```python
from build123d import *

# Parameters (mm, degrees)
EXTRUDE_1_DEPTH     = 46
SKETCH_2_R          = 3
CUT_EXTRUDE_1_DEPTH = 10
CUT_EXTRUDE_2_DEPTH = 10
FILLET_1_R          = 10


with BuildPart() as part:
    # 草图1 → 拉伸-薄壁1 (new, symmetric)
    with BuildSketch(Plane.XY):
        with BuildLine():
            Line((-15.684450605, 22.852628588), (1.315549395, 22.852628588))
            ThreePointArc((1.315549395, 22.852628588), (3.436869738, 21.973948932), (4.315549395, 19.852628588))
            Line((4.315549395, 19.852628588), (4.315549395, -12.147371412))
            ThreePointArc((4.315549395, -12.147371412), (5.194229051, -14.268691755), (7.315549395, -15.147371412))
            Line((7.315549395, -15.147371412), (17.315549395, -15.147371412))
            Line((17.315549395, -15.147371412), (17.315549395, -17.147371412))
            Line((17.315549395, -17.147371412), (7.315549395, -17.147371412))
            ThreePointArc((7.315549395, -17.147371412), (3.780015489, -15.682905318), (2.315549395, -12.147371412))
            Line((2.315549395, -12.147371412), (2.315549395, 19.852628588))
            ThreePointArc((2.315549395, 19.852628588), (2.022656176, 20.55973537), (1.315549395, 20.852628588))
            Line((1.315549395, 20.852628588), (-15.684450605, 20.852628588))
            Line((-15.684450605, 20.852628588), (-15.684450605, 22.852628588))
        make_face()
    extrude(amount=EXTRUDE_1_DEPTH, both=True)

    # 草图2 → 切除-拉伸1 (cut)
    with BuildSketch(Plane(origin=(0, -15.147371412, 0), x_dir=(1, 0, 0), z_dir=(0, 1, 0))):
        with Locations(Location((12.315549395, -38.5, 0), (0, 0, 270))):
            Circle(SKETCH_2_R)
        with Locations(Location((12.315549395, -12.5, 0), (0, 0, 270))):
            Circle(SKETCH_2_R)
        with Locations(Location((12.315549395, 12.5, 0), (0, 0, 270))):
            Circle(SKETCH_2_R)
        with Locations(Location((12.315549395, 38.5, 0), (0, 0, 270))):
            Circle(SKETCH_2_R)
    extrude(amount=-CUT_EXTRUDE_1_DEPTH, mode=Mode.SUBTRACT)

    # 草图3 → 切除-拉伸2 (cut)
    with BuildSketch(Plane(origin=(4.315549395, 0, 0), x_dir=(0, 0, -1), z_dir=(1, 0, 0))):
        with BuildLine():
            Line((-3, -7.647371412), (-3, 13.352628588))
            ThreePointArc((-3, 13.352628588), (0, 16.352628588), (3, 13.352628588))
            Line((3, 13.352628588), (3, -7.647371412))
            ThreePointArc((3, -7.647371412), (0, -10.647371412), (-3, -7.647371412))
        make_face()
    extrude(amount=-CUT_EXTRUDE_2_DEPTH, mode=Mode.SUBTRACT)

    # 圆角1
    fillet_1_edges = [part.edges().sort_by_distance(p)[0] for p in [
        (-15.684450605, 21.852628588, -46),
        (-15.684450605, 21.852628588, 46),
    ]]
    fillet(fillet_1_edges, radius=FILLET_1_R)


solid = part.part
```
CAD build for the part. Positions are in the model's coordinates, mm. A direction names the side the tool comes from. Round coordinates to 2 decimals unless told otherwise and drop trailing zeros. Order: outer loops, then holes, each group sorted by start corner. A loop starts at its lowest first (then second) coordinate and runs counter-clockwise, first axis right, second up.
Q1. Two-plate mould, pull along Z, no slides. Class faces 4 (the flat face through (12, -15.147, 1)), 5 (the cylindrical face through (-12.833, 21.867, 42.993)), 6 (the cylindrical face through (3.33, 16.35, 0.07)), 7 (the flat face through (3, 3, -3)): pulls with the +Z half, pulls with the -Z half, needs draft (parallel to the pull), parting line crosses it, or undercut.
Q2. Slice it at D-D (y = 17.5). Write the cut outline in (x, z).
Q3. Slice it at A-A (z = 12.5). Write the cut outline in (x, y).
Q4. Slice it at B-B (y = -0.5). Write the cut outline in (x, z), and give its area (3 significant figures).
Q5. Wall check: L1, parallel to X at y = 18.5, z = -35.5; L2, parallel to Y at x = 9, z = -34; L3, parallel to Y at x = 0.5, z = -5. Give the ranges that are in metal, low to high.
Q6. Which spindle directions (+Z, -Z, +X, -X, +Y, -Y) get a long thin tool onto all of the face, cutting with end or side? Do faces 1 (the flat face through (3, 3, 3)), 2 (the flat face through (2.316, 4, 11)), 3 (the cylindrical face through (12.4, -16.1, -41.5)). Say none if no direction does.
Q7. Drop flat-ended pins along their axis: pin 1 (13.5 mm diameter, centred on x = -3, z = 4.5, fed in from -Y); pin 2 (6 mm diameter, centred on x = 13, z = 12, fed in from +Y); pin 3 (8 mm diameter, centred on y = 15.5, z = -6.5, fed in from -X). Give the stop position or say it passes through.
Q8. Slice it at C-C (z = 0). Write the cut outline in (x, y).
Results below:
1. face 4: needs draft
1. face 5: pulls with the +Z half
1. face 6: undercut
1. face 7: undercut
2. outline: (2.32, -46) - (4.32, -46) - (4.32, 46) - (2.32, 46) - close
3. outline: (-15.68, 20.85) - (1.32, 20.85) arc R1 cw to (2.32, 19.85) - (2.32, -12.15) arc R5 ccw to (7.32, -17.15) - (9.32, -17.15) - (9.32, -15.15) - (7.32, -15.15) arc R3 cw to (4.32, -12.15) - (4.32, 19.85) arc R3 ccw to (1.32, 22.85) - (-15.68, 22.85) - close; (15.32, -17.15) - (17.32, -17.15) - (17.32, -15.15) - (15.32, -15.15) - close
4. outline: (2.32, -46) - (4.32, -46) - (4.32, -3) - (2.32, -3) - close; (2.32, 3) - (4.32, 3) - (4.32, 46) - (2.32, 46) - close
4. area: 172 mm2
5. L1: x = 2.32 to 4.32
5. L2: y = -17.15 to -15.15
5. L3: y = 20.85 to 22.85
6. face 1: +X, -X
6. face 2: +Z, -Z, -X, -Y
6. face 3: +Y, -Y
7. pin 1: stops at y = -15.65
7. pin 2: stops at y = -15.15
7. pin 3: stops at x = 2.32
8. outline: (-15.68, 20.85) - (1.32, 20.85) arc R1 cw to (2.32, 19.85) - (2.32, 16.35) - (4.32, 16.35) - (4.32, 19.85) arc R3 ccw to (1.32, 22.85) - (-15.68, 22.85) - close; (2.32, -12.15) arc R5 ccw to (7.32, -17.15) - (17.32, -17.15) - (17.32, -15.15) - (7.32, -15.15) arc R3 cw to (4.32, -12.15) - (4.32, -10.65) - (2.32, -10.65) - close
